Model file for the job. Use its own axes, mm. Face numbers are marked on the shaded views. A direction names the side the tool comes from. Round coordinates to 2 decimals unless told otherwise and drop trailing zeros. Order: outer loops, then holes, each group sorted by start corner. A loop starts at its lowest first (then second) coordinate and runs counter-clockwise, first axis right, second up. Notation, with made-up numbers: (-13, 12.5) - (40, 12.5) arc R30 ccw to (40, 34.5) - close; hole circle Ø11 at (57, 65.25). An arc over 180 degrees is marked (long way). Write item = value, one per line. Start each with the question number.
from build123d import *

# Parameters (mm, degrees)
F1_DEPTH = 9.652
F2_R     = 13.09002
F3_DEPTH = 25.4
F5_DEPTH = 9.6012
F4_R     = 10.091384
F4_R_2   = 10.048358
F4_R_3   = 10.112855
F4_R_4   = 10.396181
F6_DEPTH = 9.652
F7_R     = 6.272016
F7_R_2   = 6.127507
F7_R_3   = 6.686235
F7_R_4   = 6.957728
F8_DEPTH = 1.778


with BuildPart() as f1:
    # F0 (on Top) → F1 (new body)
    with BuildSketch(Plane.XY):
        with BuildLine():
            ThreePointArc((-15.598199, -9.505272), (-18.230297, -1.14468), (-16.664672, 7.479486))
            Line((-16.664672, 7.479486), (-41.31664, 0))
            Line((-41.31664, 0), (-15.598199, -9.505272))
        make_face()
        with BuildLine():
            ThreePointArc((16.664672, 7.479486), (17.86133, 3.824513), (18.266199, 0))
            ThreePointArc((18.266199, 0), (17.586555, -4.936305), (15.598199, -9.505272))
            Line((15.598199, -9.505272), (42.890608, 0))
            Line((42.890608, 0), (16.664672, 7.479486))
        make_face()
        with BuildLine():
            Line((0, -43.152936), (8.045985, -16.398663))
            ThreePointArc((8.045985, -16.398663), (0.43413, -18.261039), (-7.257626, -16.762484))
            Line((-7.257626, -16.762484), (0, -43.152936))
        make_face()
        with BuildLine():
            ThreePointArc((15.598199, -9.505272), (17.586555, -4.936305), (18.266199, 0))
            ThreePointArc((18.266199, 0), (17.86133, 3.824513), (16.664672, 7.479486))
            ThreePointArc((16.664672, 7.479486), (13.135527, 12.692988), (8.045985, 16.398663))
            ThreePointArc((8.045985, 16.398663), (0, 18.266199), (-8.045985, 16.398663))
            ThreePointArc((-8.045985, 16.398663), (-13.135527, 12.692988), (-16.664672, 7.479486))
            ThreePointArc((-16.664672, 7.479486), (-18.230297, -1.14468), (-15.598199, -9.505272))
            ThreePointArc((-15.598199, -9.505272), (-11.990162, -13.78006), (-7.257626, -16.762484))
            ThreePointArc((-7.257626, -16.762484), (0.43413, -18.261039), (8.045985, -16.398663))
            ThreePointArc((8.045985, -16.398663), (12.314283, -13.491199), (15.598199, -9.505272))
        make_face()
        with BuildLine():
            ThreePointArc((-8.045985, 16.398663), (0, 18.266199), (8.045985, 16.398663))
            Line((8.045985, 16.398663), (0, 38.168706))
            Line((0, 38.168706), (-8.045985, 16.398663))
        make_face()
    extrude(amount=F1_DEPTH)

    # F2 (on face) → F3 (cut)
    with BuildSketch(Plane(origin=(0, 0, 0), x_dir=(1, 0, 0), z_dir=(0, 0, -1))):
        Circle(F2_R)
    extrude(amount=-F3_DEPTH, mode=Mode.SUBTRACT)

    # F4 (on face) → F5 (join)
    with BuildSketch(Plane(origin=(0, 0, 0), x_dir=(1, 0, 0), z_dir=(0, 0, -1))):
        with BuildLine():
            Line((0, -38.168706), (3.498384, -28.703119))
            ThreePointArc((3.498384, -28.703119), (0, -28.077322), (-3.498384, -28.703119))
            Line((-3.498384, -28.703119), (0, -38.168706))
        make_face()
    extrude(amount=-F5_DEPTH)

    # F4 (on face) → F6 (join)
    with BuildSketch(Plane(origin=(0, 0, 0), x_dir=(1, 0, 0), z_dir=(0, 0, -1))):
        with Locations((0, -38.168706)):
            Circle(F4_R)
        with Locations((-41.31664, 0)):
            Circle(F4_R_2)
        with Locations((0, 43.152936)):
            Circle(F4_R_3)
        with Locations((42.890608, 0)):
            Circle(F4_R_4)
    extrude(amount=-F6_DEPTH)

    # F7 (on face) → F8 (join)
    with BuildSketch(Plane(origin=(0, 0, 0), x_dir=(1, 0, 0), z_dir=(0, 0, -1))):
        with Locations((-41.31664, 0)):
            Circle(F7_R)
        with Locations((0, -38.168706)):
            Circle(F7_R_2)
        with Locations((0, 43.152936)):
            Circle(F7_R_3)
        with Locations((42.890608, 0)):
            Circle(F7_R_4)
    extrude(amount=F8_DEPTH)


solid = f1.part
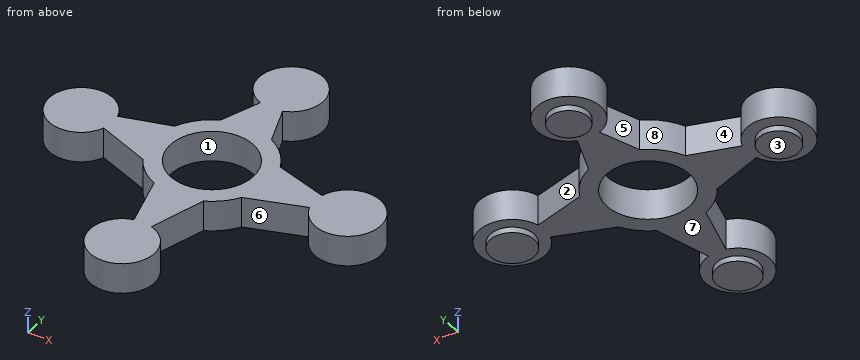
Item 1: Saw through at B-B, the plane x = 0. Give the cut face in (y, z).
Item 2: Which spindle directions (+Z, -Z, +X, -X, +Y, -Y) get a long thin tool onto all of the face, cutting with end or side? Do the marked faces 4, 5, 6, 7 and 8. Say none if no direction does.
Item 3: Drop flat-ended pins along their axis: pin 1 (8 mm diameter, centred on x = 23.5, y = -8.5, fed in from -Z); pin 2 (4 mm diameter, centred on x = 40, z = 6.5, fed in from +Y); pin 3 (3 mm diameter, centred on x = -32.5, z = 7.5, fed in from -Y). Give the stop position or say it passes through.
Item 4: Saw through at A-A, the plane y = 0. Give the cut face in (x, z) (3 decimals), then the cut area to 3 significant figures.
Item 5: Mould opens along Y. For the marked faces 1, 2 and 3 say: +Y half, -Y half, draft (parallel to the pull), parting line (faces both ways), or undercut.
Item 6: Saw through at C-C, the plane z = 4.5. Give the cut face in (x, y).
Item 7: Probe L1, parallel to X at y = 0, z = 3 (3 decimals); L2, parallel to Y at x = 0, z = 7; L3, parallel to X at y = -42, z = 6. List the from-to ranges inside material, lowest first.
Item 8: Saw through at D-D, the plane x = -18.5. Give the cut face in (y, z).
Check sheet entries:
q1.outline = (-53.27, 0) - (-49.84, 0) - (-49.84, -1.78) - (-36.47, -1.78) - (-36.47, 0) - (-13.09, 0) - (-13.09, 9.65) - (-53.27, 9.65) - close; (13.09, 0) - (32.04, 0) - (32.04, -1.78) - (44.3, -1.78) - (44.3, 0) - (48.26, 0) - (48.26, 9.65) - (13.09, 9.65) - close
q2.face_4 = +Z, -Z, +Y
q2.face_5 = +Z, -Z, -X
q2.face_6 = +Z, -Z, -Y
q2.face_7 = -Z
q2.face_8 = +Z, -Z
q3.pin_1 = 0
q3.pin_2 = 10.36
q3.pin_3 = -6.89
q4.outline = (-51.365, 0) - (-47.589, 0) - (-47.589, -1.778) - (-35.045, -1.778) - (-35.045, 0) - (-13.09, 0) - (-13.09, 9.652) - (-51.365, 9.652) - close; (13.09, 0) - (35.933, 0) - (35.933, -1.778) - (49.848, -1.778) - (49.848, 0) - (53.287, 0) - (53.287, 9.652) - (13.09, 9.652) - close
q4.area = 804 mm2
q5.face_1 = undercut
q5.face_2 = +Y half
q5.face_3 = draft
q6.outline = (-31.89, -3.48) - (-15.6, -9.51) arc R18.27 ccw to (-7.26, -16.76) - (-2.68, -33.4) arc R10.11 ccw (long way) to (2.91, -33.47) - (8.05, -16.4) arc R18.27 ccw to (15.6, -9.51) - (33.07, -3.42) arc R10.4 ccw (long way) to (32.89, 2.85) - (16.66, 7.48) arc R18.27 ccw to (8.05, 16.4) - (3.5, 28.7) arc R10.09 ccw (long way) to (-3.5, 28.7) - (-8.05, 16.4) arc R18.27 ccw to (-16.66, 7.48) - (-31.7, 2.92) arc R10.05 ccw (long way) to start; hole circle Ø26.18 at (0, 0)
q7.L1 = -51.365 to -13.09, 13.09 to 53.287
q7.L2 = -53.27 to -13.09, 13.09 to 48.26
q7.L3 = -10.05 to 10.05
q8.outline = (-8.43, 0) - (6.92, 0) - (6.92, 9.65) - (-8.43, 9.65) - close
